from build123d import *

# Parameters (mm, degrees)
SKETCH_1_R      = 25
SKETCH_1_R_2    = 11
SKETCH_1_R_3    = 2.5
SKETCH_1_R_4    = 1.65
EXTRUDE_1_DEPTH = 3


with BuildPart() as part:
    # 草图1 → 凸台-拉伸1 (new body)
    with BuildSketch(Plane.XY):
        Circle(SKETCH_1_R)
        Circle(SKETCH_1_R_2, mode=Mode.SUBTRACT)
        with Locations((10, 10)):
            Circle(SKETCH_1_R_3, mode=Mode.SUBTRACT)
        with Locations((-10, 10)):
            Circle(SKETCH_1_R_3, mode=Mode.SUBTRACT)
        with Locations((10, -10)):
            Circle(SKETCH_1_R_3, mode=Mode.SUBTRACT)
        with Locations((-10, -10)):
            Circle(SKETCH_1_R_3, mode=Mode.SUBTRACT)
        with Locations((21, 0)):
            Circle(SKETCH_1_R_4, mode=Mode.SUBTRACT)
        with Locations((-10.5, 18.186533479)):
            Circle(SKETCH_1_R_4, mode=Mode.SUBTRACT)
        with Locations((-10.5, -18.186533479)):
            Circle(SKETCH_1_R_4, mode=Mode.SUBTRACT)
    extrude(amount=EXTRUDE_1_DEPTH)


solid = part.part
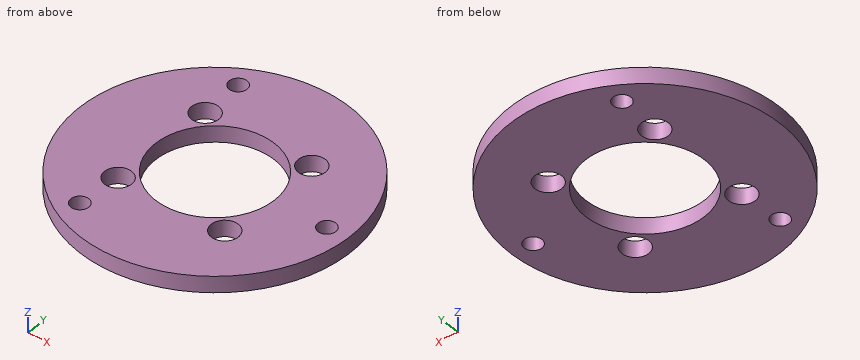
Geometry check sheet. Reference: the model listing, model coordinates, mm. Give positions to 0.01 mm unless a question says otherwise; leave off trailing zeros. Loops run counter-clockwise (first coordinate to the right, second up) from the corner with the lowest first, then second, coordinate; pieces in that order, holes last. Notation, with made-up numbers: M 22,31.25 L 38,31.25 A10 cw 38,38.25 Z; hole C -30,48 d9. An arc over 180 degrees is marked long. Answer as a JSON object with one key per item and string values. Group by question number.
Item 1: Sectioned sample at C-C on z = 0.45. Give the number of separate pieces and of enclosed holes in the cut face, plus the area to 3 significant figures.
Item 2: Material ranges on L1, parallel to X at y = -0.5, z = 2.5 (3 decimals); L2, parallel to Y at x = -10, z = 2.5; L3, parallel to Y at x = 10, z = 1.5, recorded low to high.
Item 3: Sectioned sample at D-D on x = 10. Record the boundary of the cut face in (y, z), plus the area to 3 significant figures.
Item 4: Sectioned sample at B-B on x = -6. Record the boundary of the cut face in (y, z).
Item 5: Gauge pin test, flat ends, axial feed: pin 1 (2 mm diameter, centred on x = -10.5, y = 18.19, fed in from +Z); pin 2 (6.5 mm diameter, centred on x = -10, y = -10, fed in from +Z). Record the tip position at first contact, or that the pin passes through.
Item 6: Sectioned sample at A-A on y = 0. Record the boundary of the cut face in (x, z).
Findings below:
{
 "1": {"separate pieces": "1", "enclosed holes": "8", "area": "1,480 mm2"},
 "2": {"L1": "-24.995 to -10.989, 10.989 to 19.428, 22.572 to 24.995", "L2": "-22.91 to -19.76, -16.61 to -12.5, -7.5 to -4.58, 4.58 to 7.5, 12.5 to 16.61, 19.76 to 22.91", "L3": "-22.91 to -12.5, -7.5 to -4.58, 4.58 to 7.5, 12.5 to 22.91"},
 "3": {"outline": "M -22.91,0 L -12.5,0 L -12.5,3 L -22.91,3 Z; M -7.5,0 L -4.58,0 L -4.58,3 L -7.5,3 Z; M 4.58,0 L 7.5,0 L 7.5,3 L 4.58,3 Z; M 12.5,0 L 22.91,0 L 22.91,3 L 12.5,3 Z", "area": "80.0 mm2"},
 "4": {"outline": "M -24.27,0 L -9.22,0 L -9.22,3 L -24.27,3 Z; M 9.22,0 L 24.27,0 L 24.27,3 L 9.22,3 Z"},
 "5": {"pin 1": "through", "pin 2": "z = 3"},
 "6": {"outline": "M -25,0 L -11,0 L -11,3 L -25,3 Z; M 11,0 L 19.35,0 L 19.35,3 L 11,3 Z; M 22.65,0 L 25,0 L 25,3 L 22.65,3 Z"}
}
